Source: CAD feature listing. Evaluate the final solid. Frame: model axes, mm. A direction names the side the tool comes from. Round coordinates to 2 decimals unless told otherwise and drop trailing zeros. Order: outer loops, then holes, each group sorted by start corner. A loop starts at its lowest first (then second) coordinate and runs counter-clockwise, first axis right, second up. Notation, with made-up numbers: (-4, 89.25) -> (12, 89.25) arc R24 cw to (12, 105.25) -> close; hole circle Ø2 at (66, 15). An arc over 180 degrees is marked (long way). Answer as CSV lines item,"result".
Autodesk Inventor part; units mm, degrees
ref_plane "YZ Plane" through (0, 0, 0) normal (1, 0, 0) x (0, 1, 0)
ref_plane "XZ Plane" through (0, 0, 0) normal (0, 1, 0) x (-1, 0, 0)
ref_plane "XY Plane" through (0, 0, 0) normal (0, 0, 1) x (1, 0, 0)
sketch "Sketch1" plane through (0, 0, 0) normal (0, 1, 0) x (-1, 0, 0)
  line L0 (0, -31.5) -> (0, 31.5) construction
  line L1 (-31.5, 0) -> (31.5, 0) construction
  line L2 (22.5, 22.5) -> (-22.5, 22.5)
  line L3 (-22.5, 22.5) -> (-22.5, -22.5)
  line L4 (-22.5, -22.5) -> (22.5, -22.5)
  line L5 (22.5, -22.5) -> (22.5, 22.5)
  line L6 (20, 20) -> (-20, 20)
  line L7 (-20, 20) -> (-20, -20)
  line L8 (-20, -20) -> (20, -20)
  line L9 (20, -20) -> (20, 20)
  point P0 (0, 0)
  dimension "d0" = 45
  dimension "d1" = 45
  dimension "d2" = 40
  dimension "d3" = 40
extrude "Extrusion1" add sketch "Sketch1" along normal blind 100
sketch "Sketch2" plane through (0, 100, 0) normal (0, 1, 0) x (1, 0, 0)
  line L0 (-22.5, 22.5) -> (-22.5, -22.5)
  line L1 (-22.5, -22.5) -> (22.5, -22.5)
  line L2 (22.5, -22.5) -> (22.5, 22.5)
  line L3 (22.5, 22.5) -> (-22.5, 22.5)
  point P0 (0, 0)
extrude "Extrusion2" add sketch "Sketch2" along normal blind 2.5
properties part number "UQ-753-H100-40x40x100mm" material "Glass"
1. Section query C-C on z = 12.5. Return loops of the section in (x, y).
Results below:
outline,"(-22.5, 0) -> (-20, 0) -> (-20, 100) -> (20, 100) -> (20, 0) -> (22.5, 0) -> (22.5, 102.5) -> (-22.5, 102.5) -> close"
2. Mould query, pull axis Z, two halves, no side actions, for faces 1 (the flat face through (22.5, 51, 0)), 2 (the flat face through (0, 51, 22.5)), 3 (the flat face through (0, 51, -22.5)), 4 (the flat face through (-20, 49, 0)). Classes: released by +Z, released by -Z, zero draft, split by the parting line, or undercut.
Results below:
face 1,"zero draft"
face 2,"released by +Z"
face 3,"released by -Z"
face 4,"undercut"
3. Reachability of faces 5 (the flat face through (0, 102.5, 0)), 6 (the flat face through (0, 49, 20)) from +Z, -Z, +X, -X, +Y, -Y: full face, straight path, thin tool, end or side. Return the list, or none.
Results below:
face 5,"+Z, -Z, +X, -X, +Y"
face 6,"-Y"
4. Pin query (flat end, axial travel): pin 1 (1 mm diameter, centred on x = -5.5, z = 13, fed in from -Y). Return the tip coordinate at first contact, or that it passes through.
Results below:
pin 1,"y = 100"
5. Section query A-A on y = 55.5. Return loops of the section in (x, z), and give its area (3 significant figures).
Results below:
outline,"(-22.5, -22.5) -> (22.5, -22.5) -> (22.5, 22.5) -> (-22.5, 22.5) -> close; hole (-20, -20) -> (20, -20) -> (20, 20) -> (-20, 20) -> close"
area,"425 mm2"
6. Line query: L1, parallel to X at y = 18, z = 10; L2, parallel to Y at x = 15.5, z = 10.5. Output: solid intervals per line, ascending. Write a range as [from, to].
Results below:
L1,"[-22.5, -20], [20, 22.5]"
L2,"[100, 102.5]"
7. Section query B-B on x = 1.5. Return loops of the section in (y, z).
Results below:
outline,"(0, -22.5) -> (102.5, -22.5) -> (102.5, 22.5) -> (0, 22.5) -> (0, 20) -> (100, 20) -> (100, -20) -> (0, -20) -> close"
